```python
from build123d import *

# Parameters (mm, degrees)
F0_W     = 85
F0_H     = 35
F1_DEPTH = 2.5
F2_DEPTH = 11
F4_DEPTH = 11
F6_DEPTH = 2.5


with BuildPart() as f1:
    # F0 (on Top) → F1 (new body)
    with BuildSketch(Plane.XY):
        Rectangle(F0_W, F0_H)
        with BuildLine():
            ThreePointArc((-40, 10), (-38.5355339059, 13.5355339059), (-35, 15))
            Line((-35, 15), (35, 15))
            ThreePointArc((35, 15), (38.5355339059, 13.5355339059), (40, 10))
            Line((40, 10), (40, -10))
            ThreePointArc((40, -10), (38.5355339059, -13.5355339059), (35, -15))
            Line((35, -15), (-35, -15))
            ThreePointArc((-35, -15), (-38.5355339059, -13.5355339059), (-40, -10))
            Line((-40, -10), (-40, 10))
        make_face(mode=Mode.SUBTRACT)
        with BuildLine():
            Line((35, 15), (-35, 15))
            ThreePointArc((-35, 15), (-38.5355339059, 13.5355339059), (-40, 10))
            Line((-40, 10), (-40, -10))
            ThreePointArc((-40, -10), (-38.5355339059, -13.5355339059), (-35, -15))
            Line((-35, -15), (35, -15))
            ThreePointArc((35, -15), (38.5355339059, -13.5355339059), (40, -10))
            Line((40, -10), (40, 10))
            ThreePointArc((40, 10), (38.5355339059, 13.5355339059), (35, 15))
        make_face()
    extrude(amount=-F1_DEPTH)

    # F0 (on Top) → F2 (join)
    with BuildSketch(Plane.XY):
        Rectangle(F0_W, F0_H)
        with BuildLine():
            ThreePointArc((-40, 10), (-38.5355339059, 13.5355339059), (-35, 15))
            Line((-35, 15), (35, 15))
            ThreePointArc((35, 15), (38.5355339059, 13.5355339059), (40, 10))
            Line((40, 10), (40, -10))
            ThreePointArc((40, -10), (38.5355339059, -13.5355339059), (35, -15))
            Line((35, -15), (-35, -15))
            ThreePointArc((-35, -15), (-38.5355339059, -13.5355339059), (-40, -10))
            Line((-40, -10), (-40, 10))
        make_face(mode=Mode.SUBTRACT)
    extrude(amount=F2_DEPTH)

    # F3 (on face) → F4 (cut, through all)
    with BuildSketch(Plane.XY.offset(11)):
        with BuildLine():
            Line((-35, 15), (-35, 17.5))
            Line((-35, 17.5), (-42.5, 17.5))
            Line((-42.5, 17.5), (-42.5, -17.5))
            Line((-42.5, -17.5), (-35, -17.5))
            Line((-35, -17.5), (-35, -15))
            ThreePointArc((-35, -15), (-38.5355339059, -13.5355339059), (-40, -10))
            Line((-40, -10), (-40, 10))
            ThreePointArc((-40, 10), (-38.5355339059, 13.5355339059), (-35, 15))
        make_face()
    extrude(amount=-F4_DEPTH, mode=Mode.SUBTRACT)

    # F5 (on face) → F6 (join)
    with BuildSketch(Plane.XY.offset(11)):
        with BuildLine():
            Line((-35, 12.4999995357), (35, 12.4999995357))
            ThreePointArc((35, 12.4999995357), (36.7677666247, 11.7677666247), (37.4999995357, 10))
            Line((37.4999995357, 10), (37.4999995357, -10))
            ThreePointArc((37.4999995357, -10), (36.7677666247, -11.7677666247), (35, -12.4999995357))
            Line((35, -12.4999995357), (-35, -12.4999995357))
            Line((-35, -12.4999995357), (-35, -15))
            Line((-35, -15), (35, -15))
            ThreePointArc((35, -15), (38.5355339059, -13.5355339059), (40, -10))
            Line((40, -10), (40, 10))
            ThreePointArc((40, 10), (38.5355339059, 13.5355339059), (35, 15))
            Line((35, 15), (-35, 15))
            Line((-35, 15), (-35, 12.4999995357))
        make_face()
        with BuildLine():
            Line((-35, 17.5), (-35, 15))
            Line((-35, 15), (35, 15))
            ThreePointArc((35, 15), (38.5355339059, 13.5355339059), (40, 10))
            Line((40, 10), (40, -10))
            ThreePointArc((40, -10), (38.5355339059, -13.5355339059), (35, -15))
            Line((35, -15), (-35, -15))
            Line((-35, -15), (-35, -17.5))
            Line((-35, -17.5), (42.5, -17.5))
            Line((42.5, -17.5), (42.5, 17.5))
            Line((42.5, 17.5), (-35, 17.5))
        make_face()
    extrude(amount=F6_DEPTH)


solid = f1.part
```
Geometry check sheet. Reference: the model listing, model coordinates, mm. A direction names the side the tool comes from. Give positions to 0.01 mm unless a question says otherwise; leave off trailing zeros. Order: outer loops, then holes, each group sorted by start corner. A loop starts at its lowest first (then second) coordinate and runs counter-clockwise, first axis right, second up. Notation, with made-up numbers: (-17.75, -19.75) - (23.25, -19.75) arc R15 cw to (23.25, 1.25) - close; hole circle Ø5 at (9, 86.25). An arc over 180 degrees is marked (long way). Write item = value, one per line. Start each with the question number.
1) Gauge pin test, flat ends, axial feed: pin 1 Ø5 at (x, y) = (18, 0) entering from +Z; pin 2 Ø3.5 at (y, z) = (-5, 4.5) entering from -X; pin 3 Ø2.5 at (y, z) = (15.5, 5) entering from -X. Record the tip position at first contact, or that the pin passes through.
2) Section check A-A (z = 7.25). Enter the section's corners in (x, y), then the cut area to 3 significant figures.
3) Access from +Z, -Z, +X, -X, +Y, -Y to the whole of each face (thin tool, end or side, straight path). Record for faces 1 (the cylindrical face through (38, 14, 5)), 2 (the flat face through (-35, 16, 8)), 3 (the flat face through (37.5, 0, 12)), 4 (the flat face through (-1, 0, -2.5)).
4) Section check C-C (y = -1.5). Enter the section's corners in (x, z), then the cut area to 4 significant figures.
5) Section check D-D (z = 12.5). Enter the section's corners in (x, y), then the cut area to 3 significant figures.
6) Section check B-B (x = -11). Enter the section's corners in (y, z), then the cut area to 4 significant figures.
7) Draft check along Z on faces 5 (the flat face through (6, 13, 13.5)), 6 (the flat face through (1, 17.5, 5)), 7 (the cylindrical face through (39, -13, 5)). Enter one of: released by +Z, released by -Z, zero draft, split by the parting line, or undercut.
8) Scan lines: L1, parallel to Y at x = 18, z = 8.25; L2, parallel to Z at x = 16, y = 13.5; L3, parallel to Y at x = -26, z = 13. Record each from-to range of solid material in increasing order.
Geometry check:
q1.pin_1 = 0
q1.pin_2 = 40
q1.pin_3 = -35
q2.outline = (-35, -17.5) - (42.5, -17.5) - (42.5, 17.5) - (-35, 17.5) - (-35, 15) - (35, 15) arc R5 cw to (40, 10) - (40, -10) arc R5 cw to (35, -15) - (-35, -15) - close
q2.area = 473 mm2
q3.face_1 = -X
q3.face_2 = +Z, -X, +Y, -Y
q3.face_3 = +Z, -X
q3.face_4 = -Z, +X, -X, +Y, -Y
q4.outline = (-42.5, -2.5) - (42.5, -2.5) - (42.5, 13.5) - (37.5, 13.5) - (37.5, 11) - (40, 11) - (40, 0) - (-42.5, 0) - close
q4.area = 252.5 mm2
q5.outline = (-35, -17.5) - (42.5, -17.5) - (42.5, 17.5) - (-35, 17.5) - (-35, 12.5) - (35, 12.5) arc R2.5 cw to (37.5, 10) - (37.5, -10) arc R2.5 cw to (35, -12.5) - (-35, -12.5) - close
q5.area = 903 mm2
q6.outline = (-17.5, -2.5) - (17.5, -2.5) - (17.5, 13.5) - (12.5, 13.5) - (12.5, 11) - (15, 11) - (15, 0) - (-15, 0) - (-15, 11) - (-12.5, 11) - (-12.5, 13.5) - (-17.5, 13.5) - close
q6.area = 167.5 mm2
q7.face_5 = released by +Z
q7.face_6 = zero draft
q7.face_7 = undercut
q8.L1 = -17.5 to -15, 15 to 17.5
q8.L2 = -2.5 to 0, 11 to 13.5
q8.L3 = -17.5 to -12.5, 12.5 to 17.5
